from build123d import *

# Parameters (mm, degrees)
F1_DEPTH    = 203.2
F2_T1_DEPTH = 203.2
F2_T3_DEPTH = 240.7671066227
F2_T5_DEPTH = 240.7671066227


# Not quite as in the source:
# - a fillet or chamfer that OpenCascade refuses, or shapes differently, is made with other operations: its cross-section is extruded or revolved along the edge and cut away or added


with BuildPart() as f1:
    # F0 (on Front) → F1 (new body)
    with BuildSketch(Plane.XZ):
        Polygon((-203.2, 0), (0, 0), (0, 127), (-6.35, 127), (-6.35, 6.35), (-203.2, 6.35), align=None)
    extrude(amount=F1_DEPTH)

    # F2: fillet of radius 7.62 on 3 edges, made by hand

    # F2_s2 → F2_t1 (join)
    with BuildSketch(Plane.XZ):
        with BuildLine():
            ThreePointArc((-13.97, 6.35), (-8.5818463274, 8.5818463274), (-6.35, 13.97))
            Line((-6.35, 13.97), (-6.35, 6.35))
            Line((-6.35, 6.35), (-13.97, 6.35))
        make_face()
    extrude(amount=F2_T1_DEPTH)

    # F2_s4 → F2_t3 (cut)
    with BuildSketch(Plane.XZ.offset(-18.7835533113)):
        with BuildLine():
            ThreePointArc((-195.6865786755, 6.35), (-200.6052675251, 4.5498711326), (-203.2, 0))
            Line((-203.2, 0), (-203.2, 6.35))
            Line((-203.2, 6.35), (-195.6865786755, 6.35))
        make_face()
    extrude(amount=F2_T3_DEPTH, mode=Mode.SUBTRACT)

    # F2_s6 → F2_t5 (cut)
    with BuildSketch(Plane.XZ.offset(-18.7835533113)):
        with BuildLine():
            ThreePointArc((-6.35, 119.4865786755), (-4.5498711326, 124.4052675251), (0, 127))
            Line((0, 127), (-6.35, 127))
            Line((-6.35, 127), (-6.35, 119.4865786755))
        make_face()
    extrude(amount=F2_T5_DEPTH, mode=Mode.SUBTRACT)


solid = f1.part
Verification items for the finished model (mm, model axes). A direction names the side the tool comes from. Give positions to 0.01 mm unless a question says otherwise; leave off trailing zeros. Loops run counter-clockwise (first coordinate to the right, second up) from the corner with the lowest first, then second, coordinate; pieces in that order, holes last.
1. Cross-section at C-C on x = -110. Record the cut outline in (y, z).
Derived:
outline: (-203.2, 0) - (0, 0) - (0, 6.35) - (-203.2, 6.35) - close
2. Go/stop test with flat-tipped pins: P1, Ø10, axis at x = -154.5, y = -124.5, coming from the +Z side; P2, Ø8, axis at y = -72, z = 33, coming from the -X side. Record where each tip stops, or that it passes through.
Derived:
P1: stops at z = 6.35
P2: stops at x = -6.35
3. Cross-section at B-B on z = 54.5. Record the cut outline in (x, y), and give its area (3 significant figures).
Derived:
outline: (-6.35, -203.2) - (0, -203.2) - (0, 0) - (-6.35, 0) - close
area: 1,290 mm2
4. Tool access check on faces 1 (the flat face through (-104, -100, 6.35)), 2 (the flat face through (-103, -100, 0)). Record the directions out of +Z, -Z, +X, -X, +Y, -Y that give a thin tool (end or side, any length) a straight path to the whole face; none if there is none.
Derived:
face 1: +Z, -X, +Y, -Y
face 2: -Z, +X, -X, +Y, -Y
5. Material ranges on probe 1 along Z at (x, y) = (-56.5, -90); probe 2 along X at (y, z) = (-155, 50); probe 3 along X at (y, z) = (-151.5, 12), recorded low to high.
Derived:
probe 1: z = 0 to 6.35
probe 2: x = -6.35 to 0
probe 3: x = -6.61 to 0
6. Cross-section at A-A on y = -23. Record the cut outline in (x, z).
Derived:
outline: (-203.2, 0) - (0, 0) - (0, 127) arc R7.62 ccw to (-6.35, 119.49) - (-6.35, 13.97) arc R7.62 cw to (-13.97, 6.35) - (-195.69, 6.35) arc R7.62 ccw to start
